Here's the drawing with two shaded views (mm, measured from the low corner). I have some questions. A direction names the side the tool comes from. Give positions to 0.01 mm unless a question says otherwise; leave off trailing zeros. Loops run counter-clockwise (first coordinate to the right, second up) from the corner with the lowest first, then second, coordinate; pieces in that order, holes last. Notation, with made-up numbers: (76.25, 49.25) -> (92.25, 49.25) arc R18 ccw to (92.25, 78.25) -> close; hole circle Ø5 at (77.5, -18.75). An arc over 180 degrees is marked (long way). Answer in a Markdown table with one row per item. Add a question column.
Item 1: If we section it at C-C (z = 50): Write out the boundary of the cut face in (x, y).
Item 2: Which directions (+Z, -Z, +X, -X, +Y, -Y) give clear straight access to the entire face, cutting with the end or side of a thin tool? Please do the marked faces 1, 2, 3 and 4.
Item 3: For P1, Ø8, axis at x = 93.5, z = 147.5, coming from the -Y side; P2, Ø1, axis at y = 149.5, z = 117.5, coming from the +X side; P3, Ø8, axis at x = 129, z = 80.5, coming from the +Y side, each with a flat end and sliding along its axis, tell me the tip position at first contact or that it passes through.
Item 4: If we section it at D-D (y = 23): Write out the boundary of the cut face in (x, z).
Item 5: If we section it at A-A (x = 156): Write out the boundary of the cut face in (y, z), then the cut area to 3 significant figures.
Item 6: If I drill on line 1 (Z direction, x = 100.5, y = 43.5); line 2 (Y direction, x = 126.5, z = 152), over which ranges is the centre line in solid material (lowest first)?
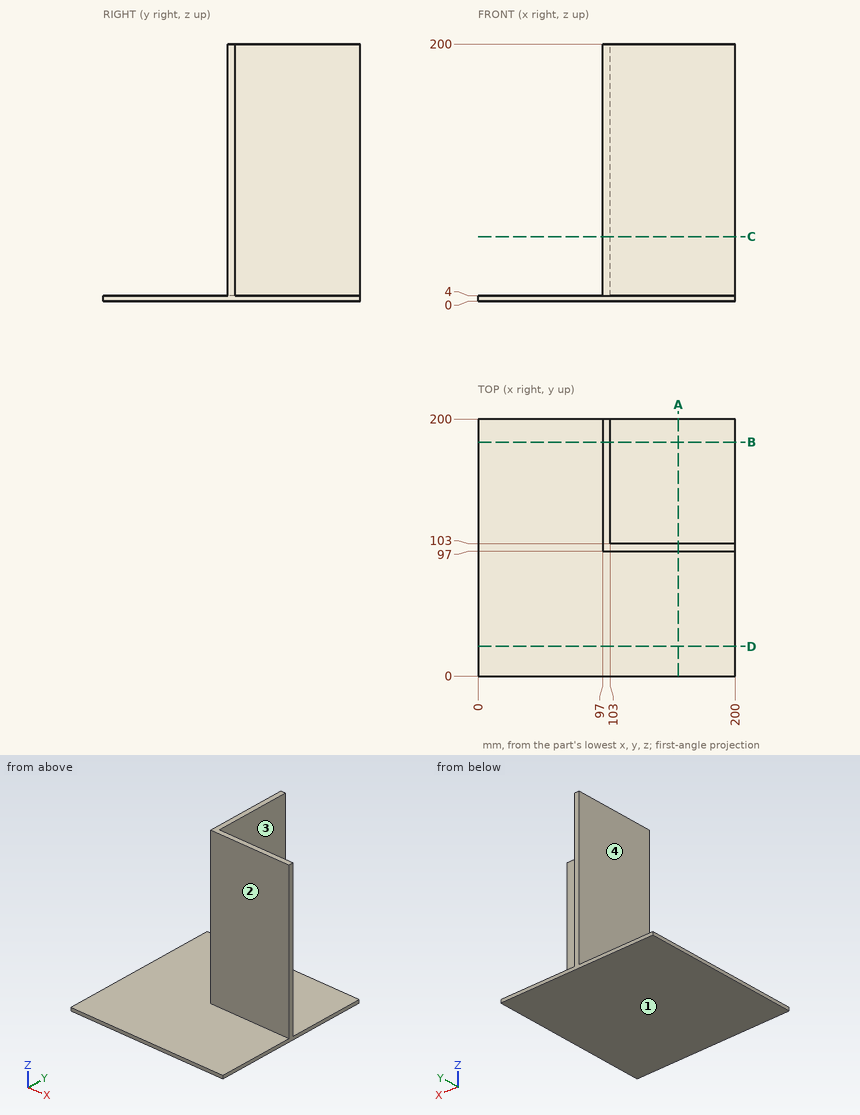
Recorded:
| question | item | result |
|---|---|---|
| 1 | outline | (97, 97) -> (200, 97) -> (200, 103) -> (103, 103) -> (103, 200) -> (97, 200) -> close |
| 2 | face 1 | -Z, +X, -X, +Y, -Y |
| 2 | face 2 | +Z, +X, -X, -Y |
| 2 | face 3 | +Z, +X, +Y |
| 2 | face 4 | +Z, -X, +Y, -Y |
| 3 | P1 | stops at y = 97 |
| 3 | P2 | stops at x = 103 |
| 3 | P3 | stops at y = 103 |
| 4 | outline | (0, 0) -> (200, 0) -> (200, 4) -> (0, 4) -> close |
| 5 | outline | (0, 0) -> (200, 0) -> (200, 4) -> (103, 4) -> (103, 200) -> (97, 200) -> (97, 4) -> (0, 4) -> close |
| 5 | area | 1,980 mm^2 |
| 6 | line 1 | z = 0 to 4 |
| 6 | line 2 | y = 97 to 103 |
